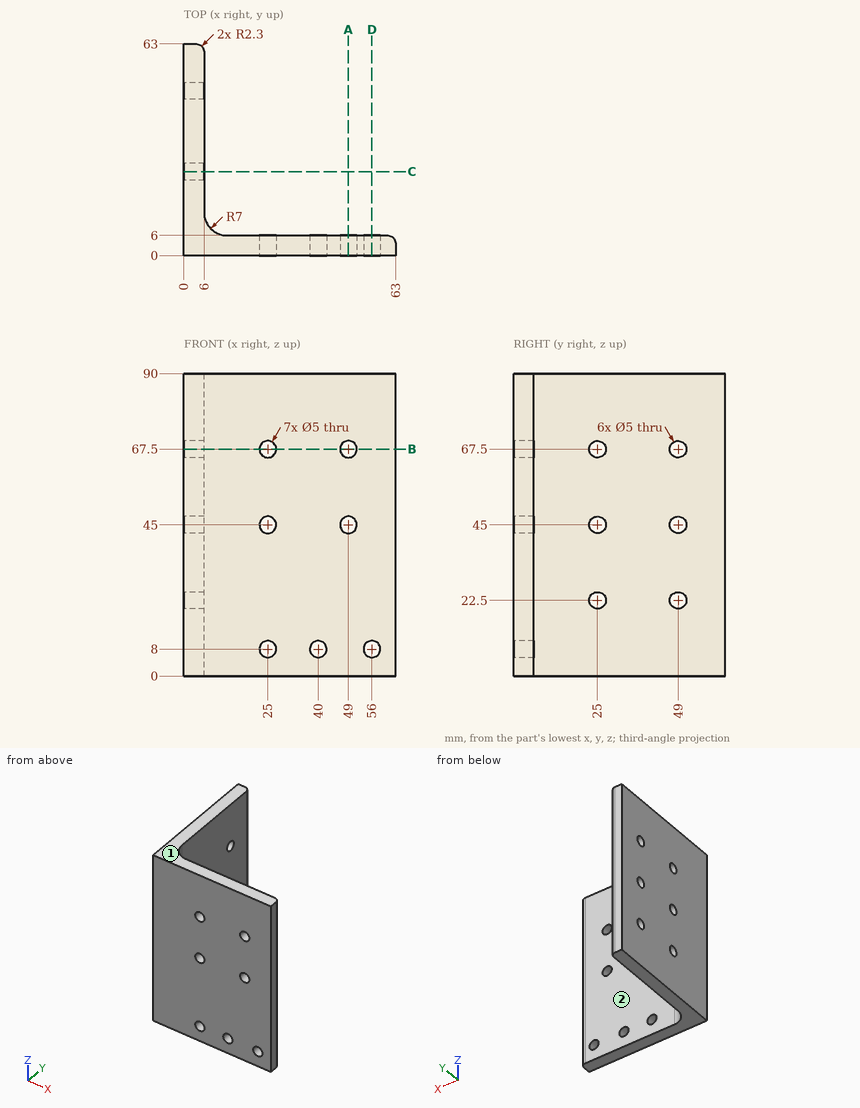
The figure shows three views and two pictorial views of one solid part (mm, origin at its lowest corner). Answer the questions. A direction names the side the tool comes from. Round coordinates to 2 decimals unless told otherwise and drop trailing zeros. Loops run counter-clockwise (first coordinate to the right, second up) from the corner with the lowest first, then second, coordinate; pieces in that order, holes last. Notation, with made-up numbers: (-17.75, -16.75) - (20.25, -16.75) arc R13 cw to (20.25, -9.75) - close; hole circle Ø10 at (17.5, 10.25). An arc over 180 degrees is marked (long way). One line per question, with ' | ' between items. Start each with the question number.
Q1. Section D-D on x = 56 is taken. Give the vertices of the cut face in (y, z), plus the area to 3 significant figures.
Q2. Section A-A on x = 49 is taken. Give the vertices of the cut face in (y, z).
Q3. For the marked faces 1 and 2, determine the directions among +Z, -Z, +X, -X, +Y, -Y from which every point of the face is accessible in a straight line to the end or side of a thin tool.
Q4. Find the intervals of material crossed by L1, parallel to Z at x = 3.4, y = 49; L2, parallel to X at y = 1.8, z = 8; L3, parallel to X at y = 2.6, z = 45, in increasing order.
Q5. Section B-B on z = 67.5 is taken. Give the vertices of the cut face in (x, y), plus the area to 3 significant figures.
Q6. Flat-ended cylindrical pins translate along their axes: pin 1 (1.5 mm diameter, centred on x = 41.5, z = 15, fed in from +Y); pin 2 (6.5 mm diameter, centred on y = 25, z = 45, fed in from +X). Find the tip coordinate at first contact, or state that the pin passes through.
Q7. Section C-C on y = 25 is taken. Give the vertices of the cut face in (x, z), plus the area to 3 significant figures.
Established:
1) outline: (0, 0) - (6, 0) - (6, 5.5) - (0, 5.5) - close; (0, 10.5) - (6, 10.5) - (6, 90) - (0, 90) - close | area: 510 mm²
2) outline: (0, 0) - (6, 0) - (6, 42.5) - (0, 42.5) - close; (0, 47.5) - (6, 47.5) - (6, 65) - (0, 65) - close; (0, 70) - (6, 70) - (6, 90) - (0, 90) - close
3) face 1: +Z, +X, -X, +Y, -Y | face 2: +Z, -Z, +X, +Y
4) L1: 0 to 20, 25 to 42.5, 47.5 to 65, 70 to 90 | L2: 0 to 22.5, 27.5 to 37.5, 42.5 to 53.5, 58.5 to 63 | L3: 0 to 22.5, 27.5 to 46.5, 51.5 to 63
5) outline: (0, 0) - (22.5, 0) - (22.5, 6) - (13, 6) arc R7 cw to (6, 13) - (6, 22.5) - (0, 22.5) - close; (0, 27.5) - (6, 27.5) - (6, 46.5) - (0, 46.5) - close; (0, 51.5) - (6, 51.5) - (6, 60.7) arc R2.3 ccw to (3.7, 63) - (0, 63) - close; (27.5, 0) - (46.5, 0) - (46.5, 6) - (27.5, 6) - close; (51.5, 0) - (63, 0) - (63, 3.7) arc R2.3 ccw to (60.7, 6) - (51.5, 6) - close | area: 608 mm²
6) pin 1: y = 6 | pin 2: x = 6
7) outline: (0, 0) - (6, 0) - (6, 20) - (0, 20) - close; (0, 25) - (6, 25) - (6, 42.5) - (0, 42.5) - close; (0, 47.5) - (6, 47.5) - (6, 65) - (0, 65) - close; (0, 70) - (6, 70) - (6, 90) - (0, 90) - close | area: 450 mm²
